Part model, mm, in its own coordinate system. A direction names the side the tool comes from. Give positions to 0.01 mm unless a question says otherwise; leave off trailing zeros. Write each loop counter-clockwise with the first axis right and the second up, starting at its lowest first coordinate (ties: lowest second). Pieces come first, ordered by that corner, then holes. Notation, with made-up numbers: (52.25, -23) - (78.25, -23) arc R22 cw to (78.25, -3) - close; hole circle Ø9 at (55.5, 13.5). An arc over 180 degrees is marked (long way). Answer as a JSON object with one key per item and string values. Group by question number.
Autodesk Inventor part; units mm, degrees
ref_plane "Work Plane2" through (-70, 8, 5) normal (0, 0, 1) x (1, 0, 0)
ref_plane "YZ Plane" through (0, 0, 0) normal (1, 0, 0) x (0, 1, 0)
ref_plane "XZ Plane" through (0, 0, 0) normal (0, 1, 0) x (-1, 0, 0)
ref_plane "Work Plane1" through (0, 0, 0) normal (0, 0, 1) x (1, 0, 0)
sketch "Sketch1" plane through (0, 0, 0) normal (0, 0, 1) x (1, 0, 0)
  circle A0 centre (23.5, 33) radius 1 construction
  circle A1 centre (23.5, 43) radius 1 construction
  circle A2 centre (24, 3) radius 1 construction
  circle A3 centre (8, 3) radius 1 construction
  circle A4 centre (16, 33) radius 1 construction
  circle A5 centre (16, 43) radius 1 construction
  circle A6 centre (7.5, 43) radius 1 construction
  circle A7 centre (7.5, 33) radius 1.0474 construction
  circle A8 centre (16, 3) radius 1 construction
  line L0 (32, 0) -> (0, 0) construction
  line L1 (32, 0) -> (32, 48) construction
  line L2 (0, 48) -> (32, 48) construction
  line L3 (0, 0) -> (0, 48) construction
  line L4 (7.5277, 79) -> (26, 79) construction
  line L5 (26, 78) -> (7.5277, 78) construction
  line L6 (32, 0) -> (0, 0)
  line L7 (0, 0) -> (0, 79)
  line L8 (0, 79) -> (32, 79)
  line L9 (32, 79) -> (32, 0)
ref_plane "Work Plane2" through (-70, 8, 5) normal (0, 0, 1) x (1, 0, 0)
extrude "Extrusion1" add sketch "Sketch1" along normal up to surface (5 mm away)
ref_plane "Work Plane3" through (-40, 38, 5) normal (0, 0, 1) x (0, 1, 0)
sketch "Sketch2" plane through (-40, 38, 5) normal (0, 0, 1) x (0, 1, 0)
  line L0 (28, 30) -> (30, 28) construction
  line L1 (28, 30) -> (-28, 30) construction
  line L2 (-30, 28) -> (-28, 30) construction
  line L3 (-30, 28) -> (-30, -28) construction
  line L4 (-28, -30) -> (-30, -28) construction
  line L5 (-28, -30) -> (28, -30) construction
  line L6 (30, -28) -> (28, -30) construction
  line L7 (30, -28) -> (30, 28) construction
  circle A0 centre (-17.5, -17.5) radius 1.95 construction
  circle A1 centre (17.5, 17.5) radius 1.95 construction
  circle A2 centre (17.5, -17.5) radius 1.95 construction
  circle A3 centre (-17.5, 17.5) radius 1.95 construction
  circle A4 centre (0, 0) radius 7.5 construction
  line L8 (-38, -40) -> (41, -40) construction
  line L9 (-38, -72) -> (-38, -40) construction
  line L10 (41, -72) -> (-38, -72) construction
  line L11 (41, -40) -> (41, -72) construction
  line L12 (41, -40) -> (-30, -40)
  line L13 (-30, -40) -> (-30, 30)
  line L14 (-30, 30) -> (41, 30)
  line L15 (41, 30) -> (41, -40)
  line L16 (41, -72) -> (-38, -72)
  line L17 (41, -40) -> (-38, -40)
  line L18 (-38, -40) -> (-38, -72)
  line L19 (-38, -72) -> (41, -72)
  line L20 (41, -72) -> (41, -40)
  point P0 (-38, -40)
  point P1 (41, -50.5)
extrude "Extrusion2" add sketch "Sketch2" along normal blind 5
sketch "Sketch3" plane through (-40, 38, 10) normal (0, 0, 1) x (1, 0, 0)
  line L0 (40, -30) -> (40, -38)
  line L1 (40, -38) -> (72, -38)
  line L2 (72, -38) -> (72, 41)
  line L3 (72, 41) -> (-30, 41)
  line L4 (-30, 41) -> (-30, -30)
  line L5 (-30, -30) -> (40, -30)
  circle A0 centre (48, -35) radius 1
  circle A1 centre (64, -35) radius 1
  circle A2 centre (63.5, 5) radius 1
  circle A3 centre (63.5, -5) radius 1
  circle A4 centre (47.5, -5) radius 1.0474
  circle A5 centre (47.5, 5) radius 1
  arc A6 (64.5499, 87.15) -> (61.0499, 90.65) centre (61.0499, 87.15) ccw
  line L6 (2.1699, 90.65) -> (61.0499, 90.65)
  arc A7 (2.1699, 90.65) -> (-1.3301, 87.15) centre (2.1699, 87.15) ccw
  line L7 (-1.3301, -52.85) -> (-1.3301, 87.15)
  arc A8 (-1.3301, -52.85) -> (2.1699, -56.35) centre (2.1699, -52.85) ccw
  line L8 (61.0499, -56.35) -> (2.1699, -56.35)
  arc A9 (61.0499, -56.35) -> (64.5499, -52.85) centre (61.0499, -52.85) ccw
  line L9 (64.5499, 87.15) -> (64.5499, -52.85)
  circle A10 centre (56, 5) radius 1
  circle A11 centre (56, -5) radius 1
  circle A12 centre (56, -35) radius 1
  point P0 (40, -38)
hole "Hole1" at (7.5, 43, 10) at (16, 43, 10) at (23.5, 43, 10) at (23.5, 33, 10) at (16, 33, 10) at (7.5, 33, 10) at (8, 3, 10) at (16, 3, 10) at (24, 3, 10) direction (0, 0, -1) diameter 3.6 depth 12 tip angle 118 counterbore diameter 6.5 counterbore depth 4
sketch "Sketch4" plane through (-40, 38, 10) normal (0, 0, 1) x (1, 0, 0)
  line L0 (20, -20) -> (-20, -20)
  circle A0 centre (-17.5, -17.5) radius 1.95
  circle A1 centre (17.5, -17.5) radius 1.95
  circle A2 centre (17.5, 17.5) radius 1.95
  circle A3 centre (-17.5, 17.5) radius 1.95
  circle A4 centre (-17.5, 17.5) radius 2.1
  point P0 (40, -38)
  dimension "d11" = 4.2
hole "Hole2" at (-57.5, 55.5, 10) at (-22.5, 55.5, 10) at (-22.5, 20.5, 10) at (-57.5, 20.5, 10) direction (0, 0, -1) diameter 4.2 depth 12 tip angle 118
sketch "Sketch5" plane through (0, 79, 0) normal (0, 1, 0) x (1, 0, 0)
  arc A0 (0.1445, 27.7) -> (-0.8555, 28.7) centre (-0.8555, 27.7) ccw construction
  line L0 (-0.8555, 28.7) -> (-4, 28.7) construction
  line L1 (-4, 28.7) -> (-4, 3) construction
  line L2 (-4, 3) -> (5.5277, 3) construction
  arc A1 (5.5277, 3) -> (6.5277, 4) centre (5.5277, 4) ccw construction
  line L3 (6.5277, 4) -> (6.5277, 5.8624) construction
  arc A2 (7.5277, 6.8624) -> (6.5277, 5.8624) centre (7.5277, 5.8624) ccw construction
  line L4 (7.5277, 6.8624) -> (26, 6.8624) construction
  line L5 (26, 6.8624) -> (26, 18.397) construction
  arc A3 (27, 19.397) -> (26, 18.397) centre (27, 18.397) ccw construction
  line L6 (27, 19.397) -> (28, 19.397) construction
  arc A4 (28, 19.397) -> (29, 20.397) centre (28, 20.397) ccw construction
  line L7 (29, 20.397) -> (29, 22.9624) construction
  arc A5 (29, 22.9624) -> (28, 23.9624) centre (28, 22.9624) ccw construction
  line L8 (28, 23.9624) -> (1.1445, 23.9624) construction
  arc A6 (0.1445, 24.9624) -> (1.1445, 23.9624) centre (1.1445, 24.9624) ccw construction
  line L9 (0.1445, 24.9624) -> (0.1445, 27.7) construction
  line L10 (8.5, 22) -> (24, 22) construction
  line L11 (24, 22) -> (24, 8.5) construction
  line L12 (24, 8.5) -> (8.5, 8.5) construction
  line L13 (8.5, 8.5) -> (8.5, 22) construction
  circle A7 centre (-1.5, 26) radius 1 construction
  circle A8 centre (5, 5.5) radius 1 construction
  circle A9 centre (26.5, 21) radius 1 construction
  line L14 (32, 0) -> (32, -10) construction
  line L15 (0, 0) -> (32, 0) construction
  line L16 (0, 0) -> (0, -5) construction
  line L17 (0, -5) -> (-70, -5) construction
  line L18 (-70, -5) -> (-70, -10) construction
  line L19 (32, -10) -> (-70, -10) construction
  line L20 (32, 0) -> (-4, 0)
  line L21 (-4, 0) -> (-4, 28.7)
  line L22 (-4, 28.7) -> (32, 28.7)
  line L23 (32, 28.7) -> (32, 0)
  line L24 (-4, 0) -> (0, 0)
  line L25 (0, 0) -> (0, -5)
  line L26 (0, -5) -> (-4, -5)
  line L27 (-4, -5) -> (-4, 0)
  line L28 (8.5, 28.7) -> (24, 28.7)
  line L29 (24, 28.7) -> (24, 8.5)
  line L30 (24, 8.5) -> (8.5, 8.5)
  line L31 (8.5, 8.5) -> (8.5, 28.7)
  circle A10 centre (5, 5.5) radius 0.75
  circle A11 centre (-1.5, 26) radius 0.75
  circle A12 centre (26.5, 21) radius 0.75
  point P0 (0, 0)
  dimension "d19" = 1.5
  dimension "d20" = 1.5
  dimension "d21" = 1.5
extrude "Extrusion3" add sketch "Sketch5" against normal blind 6 contours L20 L21 L22 L31 L30 L29 L23 | L25 L26 L27 L20
sketch "Sketch6" plane through (-70, 8, 5) normal (-1, 0, 0) x (0, 0, 1)
  circle A0 centre (61, 30) radius 1.95
  circle A1 centre (36, 55) radius 1.95
  circle A2 centre (11, 55) radius 1.95
  circle A3 centre (61, 5) radius 1.95
  circle A4 centre (11, 5) radius 1.95
  circle A5 centre (61, 55) radius 1.95
  circle A6 centre (36, 5) radius 1.95
  circle A7 centre (11, 30) radius 1.95
  line L0 (66, 58) -> (64, 60)
  line L1 (64, 60) -> (8, 60)
  line L2 (8, 60) -> (6, 58)
  line L3 (6, 58) -> (6, 2)
  line L4 (6, 2) -> (8, 0)
  line L5 (8, 0) -> (64, 0)
  line L6 (64, 0) -> (66, 2)
  line L7 (66, 2) -> (66, 58)
  line L8 (0, 71) -> (0, 0)
  line L9 (0, 0) -> (5, 0)
  line L10 (5, 71) -> (5, 0)
  line L11 (0, 71) -> (5, 71)
  line L12 (66, 0) -> (0, 0)
  line L13 (0, 0) -> (0, 71)
  line L14 (0, 71) -> (66, 71)
  line L15 (66, 71) -> (66, 0)
  point P0 (-5, -8)
extrude "Extrusion4" add sketch "Sketch6" along normal blind 6
sketch "Sketch7" plane through (-4, 79, -28.7) normal (0, 1, 0) x (1, 0, 0)
  circle A0 centre (9, -23.2) radius 0.75
  circle A1 centre (2.5, -2.7) radius 0.75
  circle A2 centre (30.5, -7.7) radius 0.75
  line L0 (36, -38.7) -> (36, 0)
  line L1 (36, 0) -> (28, 0)
  line L2 (28, 0) -> (28, -20.2)
  line L3 (28, -20.2) -> (12.5, -20.2)
  line L4 (12.5, -20.2) -> (12.5, 0)
  line L5 (12.5, 0) -> (0, 0)
  line L6 (0, 0) -> (0, -33.7)
  line L7 (0, -33.7) -> (-72, -33.7)
  line L8 (-72, -99.7) -> (-72, -33.7)
  line L9 (-66, -99.7) -> (-72, -99.7)
  line L10 (-66, -99.7) -> (-66, -38.7)
  line L11 (36, -38.7) -> (-66, -38.7)
  line L12 (-66, -99.7) -> (-72, -99.7)
  line L13 (-66, -99.7) -> (-31, -38.7)
  line L14 (-66, -38.7) -> (4, -38.7)
  line L15 (0, 0) -> (0, -33.7)
  line L16 (0, -33.7) -> (-72, -33.7)
  line L17 (-28.1311, -33.7) -> (0, -33.7)
  line L18 (0, -33.7) -> (0, 0)
  line L19 (-37.7992, -33.7) -> (-28.1311, -33.7)
  line L20 (0, -33.7) -> (0, 0)
  line L21 (0, 0) -> (-7.7257, -10.1)
  line L22 (-7.7257, -10.1) -> (-37.7992, -33.7)
  point P0 (4, -28.7)
extrude "Extrusion5" add sketch "Sketch7" against normal blind 6 contours A0 | A1 | A2 | L11 L10 L9 L8 L7 L6 L5 L4 L3 L2 L1 L0 | L13 L10 L11 | L6 L7 L22 L21
sketch "Sketch8" plane through (-40, 38, 10) normal (0, 0, 1) x (1, 0, 0)
  line L0 (0, 28) -> (-10, 28) construction
  line L1 (0, -28) -> (0, 28) construction
  line L2 (-10, -28) -> (0, -28) construction
  line L3 (-10, -28) -> (-10, 28) construction
  line L4 (-10, -28) -> (-10, 28) construction
  line L5 (-10, -28) -> (-20, -28) construction
  line L6 (-20, 28) -> (-20, -28) construction
  line L7 (-10, 28) -> (-20, 28) construction
  circle A0 centre (-17.5, -17.5) radius 2.1
  circle A1 centre (-17.5, 17.5) radius 2.1
  circle A2 centre (-17.5, -17.5) radius 5.1
  circle A3 centre (-17.5, 17.5) radius 5.1
  point P0 (40, -38)
  dimension "d28" = 3
  dimension "d29" = 3
extrude "Extrusion6" cut sketch "Sketch8" against normal blind 4 contours A1 | A2 | A3
sketch "Sketch9" plane through (-40, 38, 10) normal (0, 0, 1) x (1, 0, 0)
  line L0 (-29.973, -22.5) -> (-7.973, -22.5) construction
  line L1 (-7.973, -22.5) -> (-7.973, 23.5) construction
  line L2 (-7.973, 23.5) -> (-29.973, 23.5) construction
  line L3 (-29.973, 23.5) -> (-29.973, -22.5) construction
  line L4 (-30, -30) -> (40, -30) construction
  line L5 (-7.973, -22.5) -> (-25.973, -22.5)
  line L6 (-25.973, -22.5) -> (-25.973, 23.5)
  line L7 (-25.973, 23.5) -> (-7.973, 23.5)
  line L8 (-7.973, 23.5) -> (-7.973, -22.5)
  point P0 (40, -38)
  dimension "d32" = 22
  dimension "d33" = 46
  dimension "d34" = 7.5
  dimension "d35" = 18
extrude "Extrusion7" cut sketch "Sketch9" against normal blind 2
fillet "Fillet1" radius 12 4 edges at (-35, 76, 10) (-41.7992, 76, 5) (-11.7257, 76, -18.6) (-4, 76, -28.7)
properties part number "cellSTORM_Lasermount_v0"
1) Which spindle directions (+Z, -Z, +X, -X, +Y, -Y) get a long thin tool onto all of the face, cutting with end or side? Do faces 1 (the flat face through (16, 76, -8.5)), 2 (the flat face through (-58, 53, 6)), 3 (the flat face through (-8, 39, 10)). Say none if no direction does.
2) Band-saw the part on C-C (y = 55.5). List the corners of the cut face in (x, z), plus the area to 3 significant figures.
3) Mould opens along X. For faces 4 (the cylindrical face through (-72.96, 38.75, 67.8)), 5 (the flat face through (-57, 39, 8)), 6 (the flat face through (-76, 44, 38)) say: pulls with the +X half, pulls with the -X half, needs draft (parallel to the pull), parting line crosses it, or undercut.
4) Band-saw the part on D-D (x = -41.5). List the corners of the cut face in (y, z).
5) Probe line 1 (Y direction, x = 16, z = 2.95); line 2 (Y direction, x = 23, z = 8); line 3 (X direction, y = 20.5, z = 8.65). List the from-to ranges inside material, lowest first.
6) Drop flat-ended pins along their axis: P1, Ø6, axis at x = 7.5, y = 33, coming from the +Z side; P2, Ø10, axis at x = -50.5, y = 19, coming from the -Z side; P3, Ø4.5, axis at y = 63, z = 41, coming from the +X side; P4, Ø4, axis at x = -22.5, y = 20.5, coming from the +Z side. Give the stop position or say it passes through.
7) Band-saw the part on A-A (y = 38). List the corners of the cut face in (x, z), plus the area to 3 significant figures.
8) Band-saw the part on B-B (z = -12). List the corners of the cut face in (x, y), plus the area to 3 significant figures.
Verdict:
{
 "1": {"face 1": "-Z, +Y, -Y", "face 2": "+Z", "face 3": "+Z, +X, -Y"},
 "2": {"outline": "(-76, 5) - (-59.6, 5) - (-59.6, 6) - (-62.6, 6) - (-62.6, 8) - (-65.97, 8) - (-65.97, 10) - (-70, 10) - (-70, 71) - (-76, 71) - close; (-55.4, 5) - (-24.6, 5) - (-24.6, 10) - (-47.97, 10) - (-47.97, 8) - (-52.4, 8) - (-52.4, 6) - (-55.4, 6) - close; (-20.4, 5) - (0, 5) - (0, 0) - (32, 0) - (32, 10) - (-20.4, 10) - close", "area": "984 mm2"},
 "3": {"face 4": "needs draft", "face 5": "undercut", "face 6": "pulls with the -X half"},
 "4": {"outline": "(8, 5) - (73, 5) - (73, 4.15) - (79, 4.15) - (79, 21.33) - (73, 21.33) - (73, 10) - (8, 10) - close"},
 "5": {"line 1": "0 to 1.2, 4.8 to 31.2, 34.8 to 41.2, 44.8 to 79", "line 2": "6.09 to 29.79, 36.21 to 39.79, 46.21 to 79", "line 3": "-76 to -65.97, -47.97 to -24.6, -20.4 to 32"},
 "6": {"P1": "z = 6", "P2": "z = 5", "P3": "x = -70", "P4": "through"},
 "7": {"outline": "(-76, 5) - (0, 5) - (0, 0) - (32, 0) - (32, 10) - (-47.97, 10) - (-47.97, 8) - (-65.97, 8) - (-65.97, 10) - (-70, 10) - (-70, 14.05) - (-76, 14.05) - close; (-76, 17.95) - (-70, 17.95) - (-70, 64.05) - (-76, 64.05) - close; (-76, 67.95) - (-70, 67.95) - (-70, 71) - (-76, 71) - close", "area": "983 mm2"},
 "8": {"outline": "(-20.14, 73) - (8.5, 73) - (8.5, 79) - (-20.14, 79) - close; (24, 73) - (32, 73) - (32, 79) - (24, 79) - close", "area": "220 mm2"}
}
